```python
from build123d import *
from OCP.BRepFilletAPI import BRepFilletAPI_MakeChamfer

# Parameters (mm, degrees)
ESQUISSE1_W                  = 42
ESQUISSE1_H                  = 42
BOSS_EXTRU_1_DEPTH           = 47.5
ESQUISSE2_R                  = 11
BOSS_EXTRU_2_DEPTH           = 2
ESQUISSE3_R                  = 2.5
BOSS_EXTRU_3_DEPTH           = 24
TROU_TARAUD_M31_D            = 2.5
TROU_TARAUD_M31_DEPTH        = 4
TROU_TARAUD_M31_TIP          = 0.751075774
ESQUISSE6_OUTSIDE_W          = 62.59
ESQUISSE6_OUTSIDE_H          = 62.59
ESQUISSE6_OUTSIDE_R          = 26
ENL_V_MAT_EXTRU_1_DEPTH      = 57.020085684
ENL_V_MAT_EXTRU_2_DEPTH      = 57.020085684
ENL_V_MAT_EXTRU_2_DEPTH_BACK = 57.020085684
CHANFREIN1_SIZE              = 3
CHANFREIN1_SIZE2             = 4.28444402
ESQUISSE10_W                 = 26.659419434
ESQUISSE10_H                 = 26.659419434
BOSS_EXTRU_5_DEPTH           = 10
CHANFREIN2_SIZE              = 5
ESQUISSE11_OUTSIDE_W         = 63.576
ESQUISSE11_OUTSIDE_H         = 73.576
ENL_V_MAT_EXTRU_3_DEPTH      = 8
CONG_1_R                     = 4


with BuildPart() as part:
    # Esquisse1 → Boss.-Extru.1 (new body)
    with BuildSketch(Plane(origin=(0, 0, 0), x_dir=(0, 0, -1), z_dir=(1, 0, 0))):
        Rectangle(ESQUISSE1_W, ESQUISSE1_H)
    extrude(amount=BOSS_EXTRU_1_DEPTH)

    # Esquisse2 → Boss.-Extru.2 (add)
    with BuildSketch(Plane(origin=(0, 0, 0), x_dir=(0, 0, -1), z_dir=(1, 0, 0))):
        Circle(ESQUISSE2_R)
    extrude(amount=-BOSS_EXTRU_2_DEPTH)

    # Esquisse3 → Boss.-Extru.3 (add)
    with BuildSketch(Plane.ZY):
        with Locations(Location((0, 0, 0), (0, 0, 180))):
            Circle(ESQUISSE3_R)
    extrude(amount=BOSS_EXTRU_3_DEPTH)

    # Trou taraudé M31
    with Locations(Plane.ZY):
        with Locations((-15.5, 15.5), (15.5, 15.5), (-15.5, -15.5), (15.5, -15.5)):
            Hole(TROU_TARAUD_M31_D / 2, depth=TROU_TARAUD_M31_DEPTH)
            with Locations((0, 0, -(TROU_TARAUD_M31_DEPTH + TROU_TARAUD_M31_TIP / 2))):  # 118° drill point
                Cone(0, TROU_TARAUD_M31_D / 2, TROU_TARAUD_M31_TIP, mode=Mode.SUBTRACT)

    # Esquisse6 outside → Enlèv. mat.-Extru.1 (cut, through all)
    with BuildSketch(Plane(origin=(0, 0, 0), x_dir=(0, 0, -1), z_dir=(1, 0, 0))):
        Rectangle(ESQUISSE6_OUTSIDE_W, ESQUISSE6_OUTSIDE_H)
        Circle(ESQUISSE6_OUTSIDE_R, mode=Mode.SUBTRACT)
    extrude(amount=ENL_V_MAT_EXTRU_1_DEPTH, mode=Mode.SUBTRACT)

    # Esquisse7 → Enlèv. mat.-Extru.2 (cut, two sides: drawn at the far end of the back side and taken through both)
    with BuildSketch(Plane.XY.offset(-ENL_V_MAT_EXTRU_2_DEPTH_BACK)):
        Polygon((-184.216510411, 2), (-24, 2), (-9, 2), (-9, 2.5), (-9, 162.716510411), (-225.598714738, 398.856972015), (-400.815225149, 238.140461604), align=None)
    extrude(amount=ENL_V_MAT_EXTRU_2_DEPTH + ENL_V_MAT_EXTRU_2_DEPTH_BACK, mode=Mode.SUBTRACT)

    # Chanfrein1: one chamfer whose edges measure the first distance from different faces: ONE call of the kernel's chamfer builder (chamfer() names one face for all edges)
    chanfrein1_edges_1 = [part.edges().sort_by_distance(p)[0] for p in [
        (47.5, 0, 21),
    ]]
    chanfrein1_side_1 = [part.faces().sort_by_distance(p)[0] for p in [
        (23.75, 0, 21),
    ]]
    chanfrein1_edges_2 = [part.edges().sort_by_distance(p)[0] for p in [
        (47.5, -21, 0),
    ]]
    chanfrein1_side_2 = [part.faces().sort_by_distance(p)[0] for p in [
        (23.75, -21, 0),
    ]]
    chanfrein1_edges_3 = [part.edges().sort_by_distance(p)[0] for p in [
        (47.5, 0, -21),
    ]]
    chanfrein1_side_3 = [part.faces().sort_by_distance(p)[0] for p in [
        (23.75, 0, -21),
    ]]
    chanfrein1_edges_4 = [part.edges().sort_by_distance(p)[0] for p in [
        (47.5, 21, 0),
    ]]
    chanfrein1_side_4 = [part.faces().sort_by_distance(p)[0] for p in [
        (23.75, 21, 0),
    ]]
    chanfrein1_edges_5 = [part.edges().sort_by_distance(p)[0] for p in [
        (47.5, -18.384776311, 18.384776311),
    ]]
    chanfrein1_side_5 = [part.faces().sort_by_distance(p)[0] for p in [
        (23.75, -18.384776311, 18.384776311),
    ]]
    chanfrein1_edges_6 = [part.edges().sort_by_distance(p)[0] for p in [
        (47.5, 18.384776311, 18.384776311),
    ]]
    chanfrein1_side_6 = [part.faces().sort_by_distance(p)[0] for p in [
        (23.75, 18.384776311, 18.384776311),
    ]]
    chanfrein1_edges_7 = [part.edges().sort_by_distance(p)[0] for p in [
        (47.5, -18.384776311, -18.384776311),
    ]]
    chanfrein1_side_7 = [part.faces().sort_by_distance(p)[0] for p in [
        (23.75, -18.384776311, -18.384776311),
    ]]
    chanfrein1_edges_8 = [part.edges().sort_by_distance(p)[0] for p in [
        (47.5, 18.384776311, -18.384776311),
    ]]
    chanfrein1_side_8 = [part.faces().sort_by_distance(p)[0] for p in [
        (23.75, 18.384776311, -18.384776311),
    ]]
    chanfrein1 = BRepFilletAPI_MakeChamfer(part.part.solid().wrapped)
    for e in chanfrein1_edges_1:
        chanfrein1.Add(CHANFREIN1_SIZE, CHANFREIN1_SIZE2, e.wrapped, chanfrein1_side_1[0].wrapped)  # the first distance lies on this face
    for e in chanfrein1_edges_2:
        chanfrein1.Add(CHANFREIN1_SIZE, CHANFREIN1_SIZE2, e.wrapped, chanfrein1_side_2[0].wrapped)  # the first distance lies on this face
    for e in chanfrein1_edges_3:
        chanfrein1.Add(CHANFREIN1_SIZE, CHANFREIN1_SIZE2, e.wrapped, chanfrein1_side_3[0].wrapped)  # the first distance lies on this face
    for e in chanfrein1_edges_4:
        chanfrein1.Add(CHANFREIN1_SIZE, CHANFREIN1_SIZE2, e.wrapped, chanfrein1_side_4[0].wrapped)  # the first distance lies on this face
    for e in chanfrein1_edges_5:
        chanfrein1.Add(CHANFREIN1_SIZE, CHANFREIN1_SIZE2, e.wrapped, chanfrein1_side_5[0].wrapped)  # the first distance lies on this face
    for e in chanfrein1_edges_6:
        chanfrein1.Add(CHANFREIN1_SIZE, CHANFREIN1_SIZE2, e.wrapped, chanfrein1_side_6[0].wrapped)  # the first distance lies on this face
    for e in chanfrein1_edges_7:
        chanfrein1.Add(CHANFREIN1_SIZE, CHANFREIN1_SIZE2, e.wrapped, chanfrein1_side_7[0].wrapped)  # the first distance lies on this face
    for e in chanfrein1_edges_8:
        chanfrein1.Add(CHANFREIN1_SIZE, CHANFREIN1_SIZE2, e.wrapped, chanfrein1_side_8[0].wrapped)  # the first distance lies on this face
    add(Compound.cast(chanfrein1.Shape()), mode=Mode.REPLACE)

    # Esquisse10 → Boss.-Extru.5 (add)
    with BuildSketch(Plane.XZ.offset(21)):
        with Locations((29.170290283, 0)):
            Rectangle(ESQUISSE10_W, ESQUISSE10_H)
    extrude(amount=BOSS_EXTRU_5_DEPTH)

    # Chanfrein2
    chanfrein2_edges = [part.edges().sort_by_distance(p)[0] for p in [
        (42.5, -31, 0),
        (29.170290283, -31, 13.329709717),
        (29.170290283, -31, -13.329709717),
    ]]
    chamfer(chanfrein2_edges, length=CHANFREIN2_SIZE)

    # Esquisse11 outside → Enlèv. mat.-Extru.3 (cut)
    with BuildSketch(Plane.ZY.offset(-15.840580566)):
        with Locations((0, -5)):
            Rectangle(ESQUISSE11_OUTSIDE_W, ESQUISSE11_OUTSIDE_H)
        Polygon((0, 32.526911935), (-32.526911935, 0), (0, -32.526911935), (32.526911935, 0), align=None, mode=Mode.SUBTRACT)
    extrude(amount=ENL_V_MAT_EXTRU_3_DEPTH, mode=Mode.SUBTRACT)

    # Congé1
    cong_1_edges = [part.edges().sort_by_distance(p)[0] for p in [
        (11.840580566, 21, -11.526911935),
        (11.840580566, 21, 11.526911935),
        (11.840580566, 11.526911935, 21),
        (11.840580566, 11.526911935, -21),
        (11.840580566, -21, -11.526911935),
        (11.840580566, -11.526911935, -21),
        (11.840580566, -21, 11.526911935),
        (11.840580566, -11.526911935, 21),
    ]]
    fillet(cong_1_edges, radius=CONG_1_R)


solid = part.part
```
Source: CAD feature listing. Evaluate the final solid. Frame: model axes, mm. A direction names the side the tool comes from. Round coordinates to 2 decimals unless told otherwise and drop trailing zeros. Loops run counter-clockwise (first coordinate to the right, second up) from the corner with the lowest first, then second, coordinate; pieces in that order, holes last.
1. Contact query for flat-ended pins moving along their axis: pin 1 (6 mm diameter, centred on x = 3.5, z = -10.5, fed in from -Y); pin 2 (9 mm diameter, centred on y = -15.5, z = -15.5, fed in from +X); pin 3 (5.5 mm diameter, centred on x = 28, y = -24, fed in from -Z); pin 4 (9 mm diameter, centred on y = 17.5, z = -13.5, fed in from -X). Output: stop coordinate, or through.
2. Access query for faces 1 (the cylindrical face through (11.785, -20.704, 11.38)), 2 (the flat face through (7.841, 18, 17)), 3 (the cylindrical face through (2.03, -14.26, 15.66)), 4 (the flat face through (29, -23, 13.33)), 5 (the flat face through (6, -21, 0)). Directions: +Z, -Z, +X, -X, +Y, -Y. A direction counts if a zero-diameter tool reaches every point of the face in a straight line with its end or side. Return the directions, or none.
3. Ray query, L1, parallel to Y at x = 2.7, z = 15.5; L2, parallel to Z at x = 1, y = -15. Return the intervals inside material, ascending.
4. Section query A-A on x = 3. Output: boundary loops of the cut face in (y, z).
5. Mould query, pull axis X, two halves, no side actions, for faces 6 (the cylindrical face through (29.97, -18.345, 18.425)), 7 (the cylindrical face through (11.897, 11.421, -20.687)), 8 (the flat face through (11.897, 16.313, -16.214)), 9 (the flat face through (42.5, -23, 0)). Classes: released by +X, released by -X, zero draft, split by the parting line, or undercut.
6. Section query D-D on z = 0. Output: boundary loops of the cut face in (x, y), and give its area (3 significant figures).
7. Section query B-B on y = 0. Output: boundary loops of the cut face in (x, z).
8. Section query C-C on x = 18.5. Output: boundary loops of the cut face in (y, z).
Answers below:
1. pin 1: stops at y = -21
1. pin 2: stops at x = 47.5
1. pin 3: stops at z = -13.33
1. pin 4: stops at x = 0
2. face 1: +Z, -Y
2. face 2: +Z, +Y
2. face 3: -X
2. face 4: +Z, +X, -X, -Y
2. face 5: +Z, -Z, -X, -Y
3. L1: y = -20.87 to -16.75, -14.25 to 14.25, 16.75 to 20.87
3. L2: z = -21 to -16.65, -14.35 to 14.35, 16.65 to 21
4. outline: (-21, -15.33) arc R26 ccw to (-15.33, -21) - (15.33, -21) arc R26 ccw to (21, -15.33) - (21, 15.33) arc R26 ccw to (15.33, 21) - (-15.33, 21) arc R26 ccw to (-21, 15.33) - close; hole circle Ø2.5 at (-15.5, -15.5); hole circle Ø2.5 at (-15.5, 15.5); hole circle Ø2.5 at (15.5, -15.5); hole circle Ø2.5 at (15.5, 15.5)
5. face 6: zero draft
5. face 7: undercut
5. face 8: undercut
5. face 9: released by +X
6. outline: (-24, -2.5) - (-2, -2.5) - (-2, -11) - (0, -11) - (0, -21) - (15.84, -21) - (15.84, -31) - (37.5, -31) - (42.5, -26) - (42.5, -21) - (44.5, -21) - (47.5, -16.72) - (47.5, 16.72) - (44.5, 21) - (0, 21) - (0, 11) - (-2, 11) - (-2, 2.5) - (-9, 2.5) - (-9, 2) - (-24, 2) - close
6. area: 2,380 mm2
7. outline: (-24, -2.5) - (-2, -2.5) - (-2, -11) - (0, -11) - (0, -21) - (44.5, -21) - (47.5, -16.72) - (47.5, 16.72) - (44.5, 21) - (0, 21) - (0, 11) - (-2, 11) - (-2, 2.5) - (-24, 2.5) - close
8. outline: (-31, -8.33) - (-26, -13.33) - (-21, -13.33) - (-21, -15.33) arc R26 ccw to (-15.33, -21) - (15.33, -21) arc R26 ccw to (21, -15.33) - (21, 15.33) arc R26 ccw to (15.33, 21) - (-15.33, 21) arc R26 ccw to (-21, 15.33) - (-21, 13.33) - (-26, 13.33) - (-31, 8.33) - close
